Here's how the part is built. I have some questions about the finished solid (model axes, mm). A direction names the side the tool comes from. Coordinates: 2 decimals unless noted, no trailing zeros. Write each loop counter-clockwise with the first axis right and the second up, starting at its lowest first coordinate (ties: lowest second). Pieces come first, ordered by that corner, then holes. Notation, with made-up numbers: M 45.25,74 L 59.25,74 A23 ccw 59.25,98 Z; hole C 15,64 d7. An arc over 180 degrees is marked long. Use a Markdown table: item, result.
Autodesk Fusion 360 part; units mm, degrees
sketch "Sketch1" plane through (0, 0, 0) normal (0, 0, 1) x (1, 0, 0)
  line L0 (0, 0) -> (-50, 0)
  line L1 (-50, 0) -> (-50, 50)
  line L2 (-50, 50) -> (0, 50)
  line L3 (0, 50) -> (0, 0)
  line L4 (-45, 45) -> (-47.5, 45)
  line L5 (-47.5, 45) -> (-47.5, 47.5)
  line L6 (-47.5, 47.5) -> (-45, 47.5)
  line L7 (-45, 47.5) -> (-45, 45)
  line L8 (-45, 45) -> (-42.5, 45)
  line L9 (-42.5, 45) -> (-42.5, 42.5)
  line L10 (-42.5, 42.5) -> (-45, 42.5)
  line L11 (-45, 42.5) -> (-45, 45)
  line L12 (-42.5, 42.5) -> (-47.5, 42.5)
  line L13 (-47.5, 42.5) -> (-47.5, 47.5)
  line L14 (-47.5, 47.5) -> (-42.5, 47.5)
  line L15 (-42.5, 47.5) -> (-42.5, 42.5)
  line L16 (-30, 45) -> (-32.5, 45)
  line L17 (-32.5, 45) -> (-32.5, 47.5)
  line L18 (-32.5, 47.5) -> (-30, 47.5)
  line L19 (-30, 47.5) -> (-30, 45)
  line L20 (-32.5, 47.5) -> (-27.5, 47.5)
  line L21 (-27.5, 47.5) -> (-27.5, 42.5)
  line L22 (-27.5, 42.5) -> (-32.5, 42.5)
  line L23 (-32.5, 42.5) -> (-32.5, 47.5)
  line L24 (-15, 45) -> (-17.5, 45)
  line L25 (-17.5, 45) -> (-17.5, 47.5)
  line L26 (-17.5, 47.5) -> (-15, 47.5)
  line L27 (-15, 47.5) -> (-15, 45)
  line L28 (-17.5, 47.5) -> (-12.5, 47.5)
  line L29 (-12.5, 47.5) -> (-12.5, 42.5)
  line L30 (-12.5, 42.5) -> (-17.5, 42.5)
  line L31 (-17.5, 42.5) -> (-17.5, 47.5)
  line L32 (-15, 30) -> (-17.5, 30)
  line L33 (-17.5, 30) -> (-17.5, 32.5)
  line L34 (-17.5, 32.5) -> (-15, 32.5)
  line L35 (-15, 32.5) -> (-15, 30)
  line L36 (-17.5, 32.5) -> (-12.5, 32.5)
  line L37 (-12.5, 32.5) -> (-12.5, 27.5)
  line L38 (-12.5, 27.5) -> (-17.5, 27.5)
  line L39 (-17.5, 27.5) -> (-17.5, 32.5)
  line L40 (-45, 30) -> (-47.5, 30)
  line L41 (-47.5, 30) -> (-47.5, 32.5)
  line L42 (-47.5, 32.5) -> (-45, 32.5)
  line L43 (-45, 32.5) -> (-45, 30)
  line L44 (-47.5, 32.5) -> (-42.5, 32.5)
  line L45 (-42.5, 32.5) -> (-42.5, 27.5)
  line L46 (-42.5, 27.5) -> (-47.5, 27.5)
  line L47 (-47.5, 27.5) -> (-47.5, 32.5)
  line L48 (-30, 30) -> (-32.5, 30)
  line L49 (-32.5, 30) -> (-32.5, 32.5)
  line L50 (-32.5, 32.5) -> (-30, 32.5)
  line L51 (-30, 32.5) -> (-30, 30)
  line L52 (-32.5, 32.5) -> (-27.5, 32.5)
  line L53 (-27.5, 32.5) -> (-27.5, 27.5)
  line L54 (-27.5, 27.5) -> (-32.5, 27.5)
  line L55 (-32.5, 27.5) -> (-32.5, 32.5)
  line L56 (-45, 15) -> (-47.5, 15)
  line L57 (-47.5, 15) -> (-47.5, 17.5)
  line L58 (-47.5, 17.5) -> (-45, 17.5)
  line L59 (-45, 17.5) -> (-45, 15)
  line L60 (-47.5, 17.5) -> (-42.5, 17.5)
  line L61 (-42.5, 17.5) -> (-42.5, 12.5)
  line L62 (-42.5, 12.5) -> (-47.5, 12.5)
  line L63 (-47.5, 12.5) -> (-47.5, 17.5)
  line L64 (-30, 15) -> (-32.5, 15)
  line L65 (-32.5, 15) -> (-32.5, 17.5)
  line L66 (-32.5, 17.5) -> (-30, 17.5)
  line L67 (-30, 17.5) -> (-30, 15)
  line L68 (-32.5, 17.5) -> (-27.5, 17.5)
  line L69 (-27.5, 17.5) -> (-27.5, 12.5)
  line L70 (-27.5, 12.5) -> (-32.5, 12.5)
  line L71 (-32.5, 12.5) -> (-32.5, 17.5)
  line L72 (-15, 15) -> (-17.5, 15)
  line L73 (-17.5, 15) -> (-17.5, 17.5)
  line L74 (-17.5, 17.5) -> (-15, 17.5)
  line L75 (-15, 17.5) -> (-15, 15)
  line L76 (-17.5, 17.5) -> (-12.5, 17.5)
  line L77 (-12.5, 17.5) -> (-12.5, 12.5)
  line L78 (-12.5, 12.5) -> (-17.5, 12.5)
  line L79 (-17.5, 12.5) -> (-17.5, 17.5)
  point P0 (-45, 45)
  point P1 (-30, 45)
  point P2 (-15, 45)
  point P3 (-45, 30)
  point P4 (-30, 30)
  point P5 (-15, 30)
  point P6 (-15, 15)
  point P7 (-30, 15)
  point P8 (-45, 15)
  dimension "d1" = 2.5
  dimension "d2" = 2.5
  dimension "d3" = 2.5
  dimension "d4" = 5
  dimension "d5" = 5
  dimension "d6" = 2.5
  dimension "d7" = 2.5
  dimension "d8" = 5
  dimension "d9" = 5
  dimension "d10" = 2.5
  dimension "d11" = 2.5
  dimension "d12" = 5
  dimension "d13" = 5
  dimension "d14" = 2.5
  dimension "d15" = 2.5
  dimension "d16" = 5
  dimension "d17" = 5
  dimension "d18" = 2.5
  dimension "d19" = 2.5
  dimension "d20" = 5
  dimension "d21" = 5
extrude "Extrude1" add sketch "Sketch1" along normal blind 2
extrude "Extrude2" add sketch "Sketch1" along normal blind 7 contours L4 L11 L12 L13 | L4 L5 L6 L7 L13 L14 | L7 L8 L14 L15 | L8 L9 L10 L11 L12 L15 | L16 L19 L20 L21 L22 L23 | L16 L17 L18 L19 L20 L23 | L24 L27 L28 L29 L30 L31 | L24 L25 L26 L27 L28 L31 | L32 L35 L36 L37 L38 L39 | L32 L33 L34 L35 L36 L39 | L40 L43 L44 L45 L46 L47 | L40 L41 L42 L43 L44 L47 | L48 L51 L52 L53 L54 L55 | L48 L49 L50 L51 L52 L55 | L56 L59 L60 L61 L62 L63 | L56 L57 L58 L59 L60 L63 | L64 L67 L68 L69 L70 L71 | L64 L65 L66 L67 L68 L71 | L72 L75 L76 L77 L78 L79 | L72 L73 L74 L75 L76 L79
extrude "Extrude3" add 1 faces at (-50, 16.6667, 0.6667) along direction (-1, 0, 0) blind 5
extrude "Extrude4" cut 1 faces at (-18.3333, 0, 0.6667) along direction (0, 1, 0) blind 12.5
extrude "Extrude5" cut 1 faces at (-55, 25, 1.3333) along direction (1, 0, 0) blind 7.5
extrude "Extrude6" cut 1 faces at (-15.8333, 50, 0.6667) along direction (0, -1, 0) blind 2.5
extrude "Extrude7" cut 1 faces at (0, 35.8333, 0.6667) along direction (-1, 0, 0) blind 12.5
1. Which directions (+Z, -Z, +X, -X, +Y, -Y) give clear straight access to the entire face, cutting with the end or side of a thin tool? Please do faces 1 (the face through (-27.5, 15, 4)), 2 (the face through (-30, 27.5, 4)), 3 (the face through (-15, 30, 7)).
Answers follow:
| item | result |
|---|---|
| face 1 | +Z, +Y, -Y |
| face 2 | +Z, +X, -X |
| face 3 | +Z, +X, -X, +Y, -Y |
2. Suppose I cut it at A-A on z = 6.25. State how many separate pieces and enclosed holes the cut face has, and give its area (3 significant figures).
Answers follow:
| item | result |
|---|---|
| separate pieces | 9 |
| enclosed holes | 0 |
| area | 225 mm2 |
3. Suppose I cut it at B-B on y = 28.5. Write out the boundary of the cut face in (x, z).
Answers follow:
| item | result |
|---|---|
| outline | M -47.5,0 L -12.5,0 L -12.5,7 L -17.5,7 L -17.5,2 L -27.5,2 L -27.5,7 L -32.5,7 L -32.5,2 L -42.5,2 L -42.5,7 L -47.5,7 Z |
4. Suppose I cut it at D-D on y = 24. Write out the boundary of the cut face in (x, z).
Answers follow:
| item | result |
|---|---|
| outline | M -47.5,0 L -12.5,0 L -12.5,2 L -47.5,2 Z |
5. Suppose I cut it at C-C on x = -30.5. Write out the boundary of the cut face in (y, z), and give its area (3 significant figures).
Answers follow:
| item | result |
|---|---|
| outline | M 12.5,0 L 47.5,0 L 47.5,7 L 42.5,7 L 42.5,2 L 32.5,2 L 32.5,7 L 27.5,7 L 27.5,2 L 17.5,2 L 17.5,7 L 12.5,7 Z |
| area | 145 mm2 |
6. We'd pull the mould along Y, two halves only. Please class faces 4 (the face through (-15, 42.5, 4)), 5 (the face through (-45, 30, 7)), 6 (the face through (-30, 12.5, 3)): +Y half, -Y half, draft (parallel to the pull), parting line (faces both ways), or undercut.
Answers follow:
| item | result |
|---|---|
| face 4 | undercut |
| face 5 | draft |
| face 6 | -Y half |
7. I need wall thicknesses on probe 1 along X at (y, z) = (29, 4.5); probe 2 along Y at (x, z) = (-30.5, 3.75); probe 3 along Z at (x, y) = (-17, 37). Which ranges of each line are inside material? Lowest first, please.
Answers follow:
| item | result |
|---|---|
| probe 1 | x = -47.5 to -42.5, -32.5 to -27.5, -17.5 to -12.5 |
| probe 2 | y = 12.5 to 17.5, 27.5 to 32.5, 42.5 to 47.5 |
| probe 3 | z = 0 to 2 |
